from build123d import *

# Parameters (mm, degrees)
FILLET1_R           = 0.508
LPATTERN1_COUNT     = 8
LPATTERN1_PITCH     = 150
LPATTERN1_COL_COUNT = 3
LPATTERN1_COL_PITCH = 150


with BuildPart() as part:
    # Sketch1 → Revolve1 (revolve)
    with BuildSketch(Plane(origin=(0, 0, 0), x_dir=(1, 0, 0), z_dir=(0, 1, 0)), mode=Mode.PRIVATE) as revolve1_sk:
        Polygon((0, 1550), (0, -20), (1.473460386, -20), (5, 0), (10, 0), (10, 1550), align=None)
    revolve(revolve1_sk.sketch.rotate(Axis((0, 0, -1550), (0, 0, 1)), 180), axis=Axis((0, 0, -1550), (0, 0, 1)))  # turned: the seam where the file's is

    # Fillet1
    fillet1_edges = [part.edges().sort_by_distance(p)[0] for p in [
        (10, 0, -1550),
        (10, 0, 0),
        (1.473460386, 0, 20),
    ]]
    fillet(fillet1_edges, radius=FILLET1_R)

    # Sketch3 → M6x1.0 Tapped Hole1 (revolve, cut)
    with BuildSketch(Plane(origin=(0, 10, -1109.22499992), x_dir=(0, 0, 1), z_dir=(1, 0, 0))):
        Polygon((0, 0), (0, 16.502151548), (2.5, 15), (2.5, 0), align=None)
    m6x1_0_tapped_hole1 = revolve(axis=Axis((0, 16.35, -1109.22499992), (0, -1, 0)), mode=Mode.SUBTRACT)

    # LPattern1: M6x1.0 Tapped Hole1 ×8
    with Locations(*[(0, 0, i * LPATTERN1_PITCH) for i in range(1, LPATTERN1_COUNT)]):
        add(m6x1_0_tapped_hole1, mode=Mode.SUBTRACT)

    # LPattern1 col: M6x1.0 Tapped Hole1 ×3
    with Locations(*[(0, 0, -i * LPATTERN1_COL_PITCH) for i in range(1, LPATTERN1_COL_COUNT)]):
        add(m6x1_0_tapped_hole1, mode=Mode.SUBTRACT)


solid = part.part
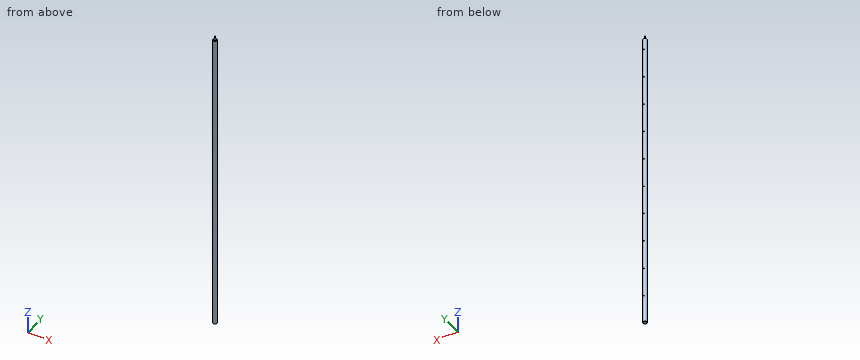
Input: part model. Units: mm. Frame: model coordinates. Give positions to 0.01 mm unless a question says otherwise; leave off trailing zeros. Order: outer loops, then holes, each group sorted by start corner. A loop starts at its lowest first (then second) coordinate and runs counter-clockwise, first axis right, second up. Notation, with made-up numbers: (12, 84.5) - (65, 84.5) arc R21 cw to (65, 104.5) - close; hole circle Ø11 at (10.5, -35). An arc over 180 degrees is marked (long way). Answer as a JSON object with one key per item and string values. Group by question number.
Q1. Line query: probe 1 along Z at (x, y) = (3.75, 7.75); probe 2 along Y at (x, z) = (1.75, -738.5); probe 3 along X at (y, z) = (-0.25, -835). Output: solid intervals per line, ascending.
Q2. Cut plane A-A, the plane z = -835.5. Output: boundary loops of the cut face in (x, y), then the cut area to 3 significant figures.
Q3. First-contact query: pin 1 Ø4 at (x, z) = (0, -359.225) entering from +Y; pin 2 Ø1 at (y, z) = (-7.5, -1379.5) entering from +X; pin 3 Ø2 at (x, z) = (3, -1170) entering from +Y. Flat tips, straight axial feed; report the tip coordinate or a pass-through.
Results:
{
 "1": {"probe 1": "-1550 to 0", "probe 2": "-9.85 to 9.85", "probe 3": "-10 to 10"},
 "2": {"outline": "circle Ø20 at (0, 0)", "area": "314 mm^2"},
 "3": {"pin 1": "y = -5.3", "pin 2": "x = 7.14", "pin 3": "y = 9.8"}
}
